Here's how the part is built. I have some questions about the finished solid (model axes, mm). Give positions to 0.01 mm unless a question says otherwise; leave off trailing zeros. Order: outer loops, then holes, each group sorted by start corner. A loop starts at its lowest first (then second) coordinate and runs counter-clockwise, first axis right, second up. Notation, with made-up numbers: M 70,-35 L 112,-35 A13 cw 112,-20 Z; hole C 28.5,68.25 d4. An arc over 180 degrees is marked long. Use CSV: the item, a comma, the result in double quotes. Start each with the question number.
```python
from build123d import *

# Parameters (mm, degrees)
SKETCH1_W                                       = 95.25
SKETCH1_H                                       = 25
SKETCH1_H_2                                     = 63.5
SKETCH1_R                                       = 14.2621
SKETCH1_R_2                                     = 3.81
BOSS_EXTRUDE1_DEPTH                             = 6.35
F_1_4_CLEARANCE_HOLE2_D                         = 6.7564
FILLET1_R                                       = 5.08
CSK_FOR_M4_FLAT_HEAD_MACHINE_SCREW2_D           = 4.5
CSK_FOR_M4_FLAT_HEAD_MACHINE_SCREW2_CSINK_D     = 9.4
CSK_FOR_M4_FLAT_HEAD_MACHINE_SCREW2_CSINK_ANGLE = 90


with BuildPart() as part:
    # Sketch1 → Boss-Extrude1 (new body)
    # profile 1 of 2: a face of its own
    with BuildSketch(Plane(origin=(0, 0, 0), x_dir=(0, 0, -1), z_dir=(1, 0, 0))):
        with Locations((-20.575, 44.25)):
            Rectangle(SKETCH1_W, SKETCH1_H)
    # profile 2 of 2: a face of its own
    with BuildSketch(Plane(origin=(0, 0, 0), x_dir=(0, 0, -1), z_dir=(1, 0, 0))):
        with Locations((-20.575, 0)):
            Rectangle(SKETCH1_W, SKETCH1_H_2)
        with Locations((-31.8887, 0)):
            Circle(SKETCH1_R, mode=Mode.SUBTRACT)
        Circle(SKETCH1_R_2, mode=Mode.SUBTRACT)
    extrude(amount=BOSS_EXTRUDE1_DEPTH)

    # 1/4 Clearance Hole2 (through all)
    with Locations(Plane(origin=(6.35, 0, 0), x_dir=(0, 0, -1), z_dir=(1, 0, 0))):
        with Locations((-55.5, 44.25), (-20.575, 44.25), (14.35, 44.25), (-61.85, -25.4), (20.7, -25.4)):
            Hole(F_1_4_CLEARANCE_HOLE2_D / 2)

    # Fillet1
    fillet1_edges = [part.edges().sort_by_distance(p)[0] for p in [
        (3.175, -31.75, -27.05),
        (3.175, -31.75, 68.2),
        (3.175, 56.75, 68.2),
        (3.175, 56.75, -27.05),
    ]]
    fillet(fillet1_edges, radius=FILLET1_R)

    # CSK for M4 Flat Head Machine Screw2 (through all)
    with Locations(Plane.ZY):
        with Locations((-8, 8), (8, 8), (8, -8), (-8, -8)):
            CounterSinkHole(CSK_FOR_M4_FLAT_HEAD_MACHINE_SCREW2_D / 2, CSK_FOR_M4_FLAT_HEAD_MACHINE_SCREW2_CSINK_D / 2, counter_sink_angle=CSK_FOR_M4_FLAT_HEAD_MACHINE_SCREW2_CSINK_ANGLE)


solid = part.part
```
Q1. Imagine slicing it at C-C, the plane y = -25.4. Please give me the cut outline in (x, z).
Q2. We'd pull the mould along Y, two halves only. Please class faces 1 (the face through (3, 12, -27.05)), 2 (the face through (3.219, -30.222, 66.751)), 3 (the face through (3.13, 40.95, -15.08)): pulls with the +Y half, pulls with the -Y half, needs draft (parallel to the pull), parting line crosses it, or undercut.
Q3. I need wall thicknesses on line 1 (Y direction, x = 5.35, z = 8); line 2 (Z direction, x = 3.5, y = -8); line 3 (Y direction, x = 3, z = 61.85). Which ranges of each line are inside material? Lowest first, please. Write a range as [from, to].
Q4. Imagine slicing it at D-D, the plane z = -14.35. Please give me the cut outline in (x, y).
Q5. Imagine slicing it at A-A, the plane z = 0. Please give me the cut outline in (x, y), then the cut area to 3 significant figures.
Q6. For P1, Ø5, axis at y = -8, z = 8, coming from the -X side; P2, Ø8, axis at y = 44.25, z = 20.575, coming from the +X side; P3, Ø7, axis at y = 8, z = -8, coming from the -X side, each with a flat end and sliding along its axis, tell me the tip position at first contact or that it passes through.
Q7. Imagine slicing it at B-B, the plane y = 44.25. Please give me the cut outline in (x, z), then the cut area to 3 significant figures.
Reply:
1,outline,"M 0,-27.05 L 6.35,-27.05 L 6.35,-24.08 L 0,-24.08 Z; M 0,-17.32 L 6.35,-17.32 L 6.35,58.47 L 0,58.47 Z; M 0,65.23 L 6.35,65.23 L 6.35,68.2 L 0,68.2 Z"
2,face 1,"needs draft"
2,face 2,"pulls with the -Y half"
2,face 3,"undercut"
3,line 1,"y = [-31.75, -10.25], [-5.75, 5.75], [10.25, 56.75]"
3,line 2,"z = [-27.05, -10.25], [-5.75, 5.75], [10.25, 20.08], [43.7, 68.2]"
3,line 3,"y = [-31.75, -28.78], [-22.02, 56.75]"
4,outline,"M 0,-31.75 L 6.35,-31.75 L 6.35,40.87 L 0,40.87 Z; M 0,47.63 L 6.35,47.63 L 6.35,56.75 L 0,56.75 Z"
5,outline,"M 0,-31.75 L 6.35,-31.75 L 6.35,-3.81 L 0,-3.81 Z; M 0,3.81 L 6.35,3.81 L 6.35,56.75 L 0,56.75 Z"
5,area,"514 mm^2"
6,P1,"stops at x = 2.2"
6,P2,"stops at x = 6.35"
6,P3,"stops at x = 1.2"
7,outline,"M 0,-27.05 L 6.35,-27.05 L 6.35,-17.73 L 0,-17.73 Z; M 0,-10.97 L 6.35,-10.97 L 6.35,17.2 L 0,17.2 Z; M 0,23.95 L 6.35,23.95 L 6.35,52.12 L 0,52.12 Z; M 0,58.88 L 6.35,58.88 L 6.35,68.2 L 0,68.2 Z"
7,area,"476 mm^2"
